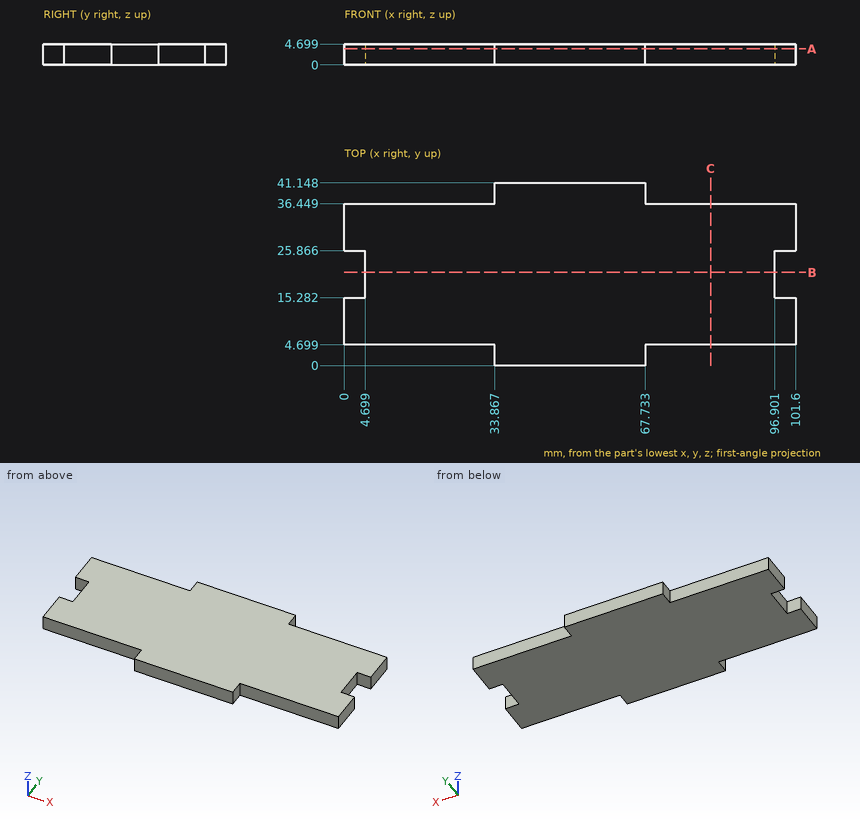
Part print with two shaded views. Sizes in mm from the minimum x, y, z corner. Round coordinates to 2 decimals unless told otherwise and drop trailing zeros. Loops run counter-clockwise (first coordinate to the right, second up) from the corner with the lowest first, then second, coordinate; pieces in that order, holes last.
1. Flat gauge pins, fed straight in: pin 1 (1.5 mm diameter, centred on y = 26.5, z = 3, fed in from -X); pin 2 (1.5 mm diameter, centred on x = 77.5, z = 3.5, fed in from -Y); pin 3 (1.4 mm diameter, centred on y = 23, z = 1.5, fed in from +X); pin 4 (1.4 mm diameter, centred on x = 15.5, z = 3, fed in from +Y). Where does each tip first touch, or does it go through?
Solutions:
pin 1: stops at x = 0
pin 2: stops at y = 4.7
pin 3: stops at x = 96.9
pin 4: stops at y = 36.45
2. Slice it at B-B (y = 21). Give the cut face in (x, z), and give its area (3 significant figures).
Solutions:
outline: (4.7, 0) - (96.9, 0) - (96.9, 4.7) - (4.7, 4.7) - close
area: 433 mm2
3. Slice it at C-C (x = 82.5). Give the cut face in (y, z), and give its area (3 significant figures).
Solutions:
outline: (4.7, 0) - (36.45, 0) - (36.45, 4.7) - (4.7, 4.7) - close
area: 149 mm2
4. Slice it at A-A (z = 3.6). Give the cut face in (x, y) (1 decimal).
Solutions:
outline: (0, 4.7) - (33.9, 4.7) - (33.9, 0) - (67.7, 0) - (67.7, 4.7) - (101.6, 4.7) - (101.6, 15.3) - (96.9, 15.3) - (96.9, 25.9) - (101.6, 25.9) - (101.6, 36.4) - (67.7, 36.4) - (67.7, 41.1) - (33.9, 41.1) - (33.9, 36.4) - (0, 36.4) - (0, 25.9) - (4.7, 25.9) - (4.7, 15.3) - (0, 15.3) - close
5. Drill centre lines: line 1 along Y through (x, z) = (78.5, 4.45); line 2 along X through (y, z) = (22, 2.8); line 3 along X through (y, z) = (2.5, 3.95). Where is each one in solid material? Low to high.
Solutions:
line 1: y = 4.7 to 36.45
line 2: x = 4.7 to 96.9
line 3: x = 33.87 to 67.73
